from build123d import *

# Parameters (mm, degrees)
F1_DEPTH = 39
F3_DEPTH = 2
F4_R     = 2.5
F5_DEPTH = 24
F6_R     = 1.5
F7_DEPTH = 5


with BuildPart() as f1:
    # F0 (on Front) → F1 (new body)
    with BuildSketch(Plane.XZ):
        Polygon((21.15, 18.15), (18.15, 21.15), (-18.15, 21.15), (-21.15, 18.15), (-21.15, -18.15), (-18.15, -21.15), (18.15, -21.15), (21.15, -18.15), align=None)
    extrude(amount=F1_DEPTH)

    # F2 (on face) → F3 (join)
    with BuildSketch(Plane.XZ.offset(39)):
        with BuildLine():
            ThreePointArc((-11, 0), (-7.7781745931, -7.7781745931), (0, -11))
            Line((0, -11), (0, 0))
            Line((0, 0), (-11, 0))
        make_face()
        with BuildLine():
            Line((0, 0), (0, 11))
            ThreePointArc((0, 11), (-7.7781745931, 7.7781745931), (-11, 0))
            Line((-11, 0), (0, 0))
        make_face()
        with BuildLine():
            Line((0, 0), (11, 0))
            ThreePointArc((11, 0), (7.7781745931, 7.7781745931), (0, 11))
            Line((0, 11), (0, 0))
        make_face()
        with BuildLine():
            ThreePointArc((0, -11), (7.7781745931, -7.7781745931), (11, 0))
            Line((11, 0), (0, 0))
            Line((0, 0), (0, -11))
        make_face()
    extrude(amount=F3_DEPTH)

    # F4 (on face) → F5 (join)
    with BuildSketch(Plane.XZ.offset(41)):
        Circle(F4_R)
    extrude(amount=F5_DEPTH)

    # F6 (on face) → F7 (cut)
    with BuildSketch(Plane.XZ.offset(39)):
        with Locations((-15.5, 15.5)):
            Circle(F6_R)
        with BuildLine():
            ThreePointArc((17, 15.5), (15.5, 17), (14, 15.5))
            ThreePointArc((14, 15.5), (15.5, 14), (17, 15.5))
        make_face()
        with Locations((15.5, -15.5)):
            Circle(F6_R)
        with Locations((-15.5, -15.5)):
            Circle(F6_R)
    extrude(amount=-F7_DEPTH, mode=Mode.SUBTRACT)


solid = f1.part
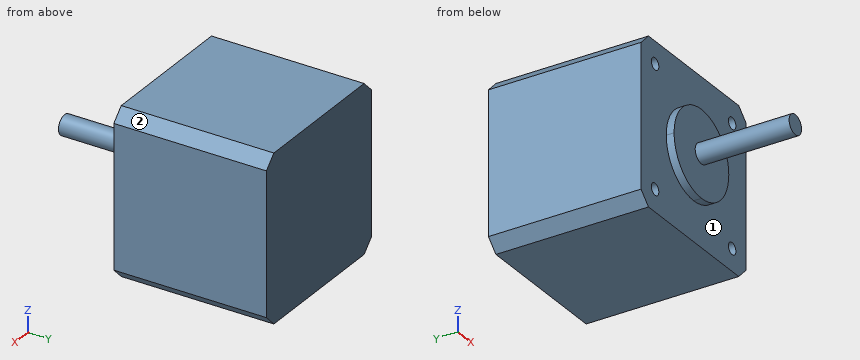
Read the model definition and answer for the solid it produces. Units are mm, in the model's axes. Face numbers are marked on the shaded views. A direction names the side the tool comes from. Coordinates: 2 decimals unless noted, no trailing zeros. Loops run counter-clockwise (first coordinate to the right, second up) from the corner with the lowest first, then second, coordinate; pieces in that order, holes last.
Q1. The part is cut by section B-B on y = -59. Write down the section's boundary in (x, z).
Q2. The part is cut by section D-D on x = 9. Write down the section's boundary in (y, z), and give its area (4 significant figures).
Q3. The part is cut by section A-A on x = 15.5. Write down the section's boundary in (y, z).
Q4. Consider probe 1 along Z at (x, y) = (-15.5, -35.8); probe 2 along X at (y, z) = (-35, 15); probe 3 along Y at (x, z) = (-3, 19). Determine where each line is inside the solid, lowest interval first.
Q5. Which of the six approach directions +Z, -Z, +X, -X, +Y, -Y give full straight-line access (tool end or side, diameter ignored) to the marked faces 1 and 2?
Q6. Each of these flat-tipped pins is pushed along its axis until it touches: pin 1 Ø0.9 at (x, z) = (15.5, 15) entering from -Y; pin 2 Ø4 at (x, y) = (1, -45) entering from +Z; pin 3 Ø3.5 at (x, z) = (15.5, 15.5) entering from -Y. Where does it stop, or does it pass through?
Q7. The part is cut by section C-C on z = -1.5. Write down the section's boundary in (x, y), and give its area (3 significant figures).
Results below:
1. outline: circle Ø5 at (0, 0)
2. outline: (-41, -6.32) - (-39, -6.32) - (-39, -21.15) - (0, -21.15) - (0, 21.15) - (-39, 21.15) - (-39, 6.32) - (-41, 6.32) - close
2. area: 1,675 mm2
3. outline: (-39, -21.15) - (0, -21.15) - (0, 21.15) - (-39, 21.15) - (-39, 17) - (-34, 17) - (-34, 14) - (-39, 14) - (-39, -14) - (-34, -14) - (-34, -17) - (-39, -17) - close
4. probe 1: z = -21.15 to -17, -14 to 14, 17 to 21.15
4. probe 2: x = -21.15 to -16.91, -14.09 to 14.09, 16.91 to 21.15
4. probe 3: y = -39 to 0
5. face 1: -Y
5. face 2: +Z, +X, +Y, -Y
6. pin 1: stops at y = -34
6. pin 2: stops at z = 2.5
6. pin 3: stops at y = -39
7. outline: (-21.15, -39) - (-10.9, -39) - (-10.9, -41) - (-2, -41) - (-2, -65) - (2, -65) - (2, -41) - (10.9, -41) - (10.9, -39) - (21.15, -39) - (21.15, 0) - (-21.15, 0) - close
7. area: 1,790 mm2
